Print and shaded views of the part. All mm, measured from the part's lowest x, y and z. Coordinates: 2 decimals unless noted, no trailing zeros. Loops run counter-clockwise (first coordinate to the right, second up) from the corner with the lowest first, then second, coordinate; pieces in that order, holes last. Notation, with made-up numbers: M -12.75,69 L 45.25,69 A12 ccw 45.25,84 Z; hole C -12.75,16.5 d7. An arc over 180 degrees is marked long. Use a Markdown table: item, result. Add a question column.
1) Band-saw the part on C-C (y = 21.5). List the corners of the cut face in (x, z), plus the area to 3 significant figures.
2) Pull direction Y, two halves, no side cores. Call the marked faces 1, 2 and 3: released by +Y, released by -Y, zero draft, split by the parting line, or undercut.
3) Band-saw the part on B-B (z = 114). List the corners of the cut face in (x, y).
4) Pin check, flat tips, straight feed: pin 1 Ø20 at (y, z) = (25, 155.5) entering from +X; pin 2 Ø3 at (y, z) = (51.5, 80.5) entering from +X; pin 3 Ø6 at (y, z) = (51, 151) entering from +X. Stop position of each tip, or through.
5) Band-saw the part on A-A (x = 32.5). List the corners of the cut face in (y, z), plus the area to 3 significant figures.
6) Wall check: probe 1 along Y at (x, z) = (34, 81); probe 2 along X at (y, z) = (18.5, 214.5); probe 3 along Y at (x, z) = (11, 45). Give the ranges that are in metal, low to high. Write a range as from..to.
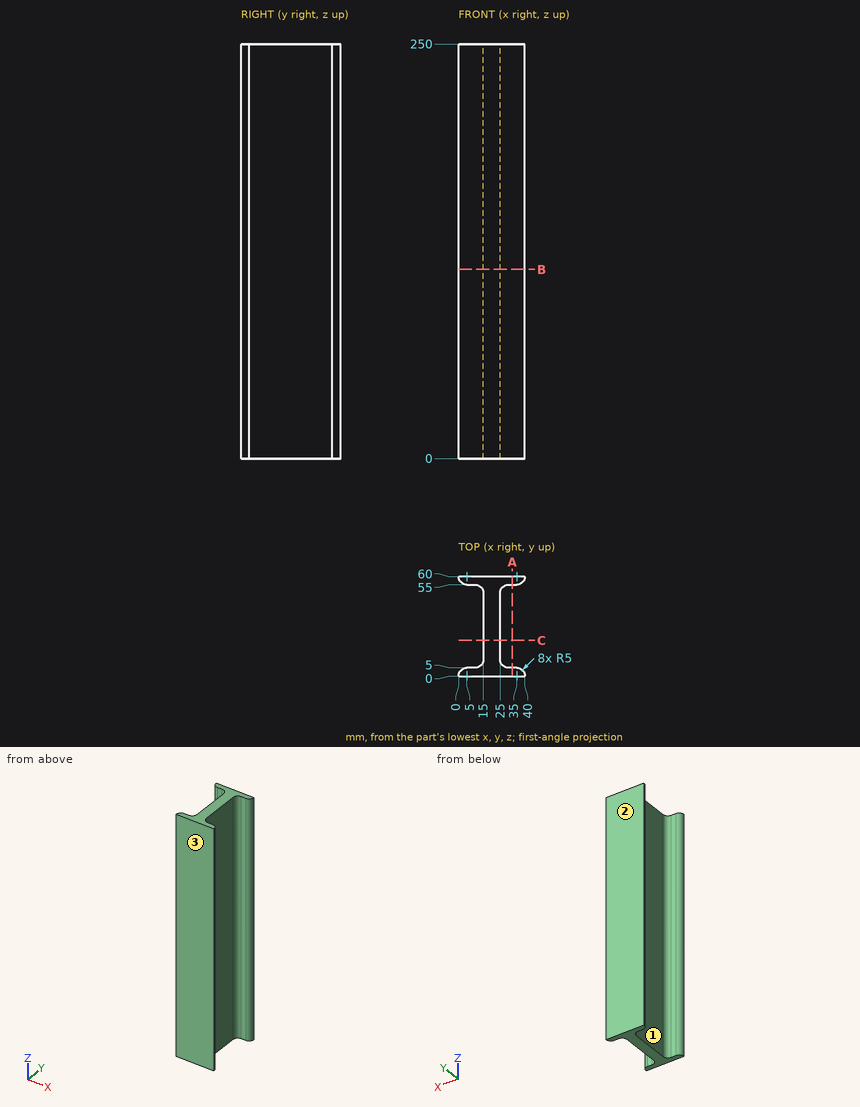
Entries:
| question | item | result |
|---|---|---|
| 1 | outline | M 15,0 L 25,0 L 25,250 L 15,250 Z |
| 1 | area | 2,500 mm2 |
| 2 | face 1 | undercut |
| 2 | face 2 | released by +Y |
| 2 | face 3 | released by -Y |
| 3 | outline | M 0,0 L 40,0 A5 ccw 35,5 L 30,5 A5 cw 25,10 L 25,50 A5 cw 30,55 L 35,55 A5 ccw 40,60 L 0,60 A5 ccw 5,55 L 10,55 A5 cw 15,50 L 15,10 A5 cw 10,5 L 5,5 A5 ccw Z |
| 4 | pin 1 | x = 25 |
| 4 | pin 2 | x = 26 |
| 4 | pin 3 | x = 27 |
| 5 | outline | M 0,0 L 5,0 L 5,250 L 0,250 Z; M 55,0 L 60,0 L 60,250 L 55,250 Z |
| 5 | area | 2,500 mm2 |
| 6 | probe 1 | 0..5, 55..60 |
| 6 | probe 2 | 15..25 |
| 6 | probe 3 | 0..5.1, 54.9..60 |
